For this review, use the dimensioned drawing (mm, ordinates from the lowest corner) and the shaded views. A direction names the side the tool comes from. Coordinates: 2 decimals unless noted, no trailing zeros. Loops run counter-clockwise (first coordinate to the right, second up) from the corner with the lowest first, then second, coordinate; pieces in that order, holes last. Notation, with made-up numbers: (58, -3.5) - (91, -3.5) arc R19 ccw to (91, 17.5) - close; hole circle Ø6 at (-4, 39). An arc over 180 degrees is marked (long way). Return JSON: item names as keys, results as strings. Group by question number.
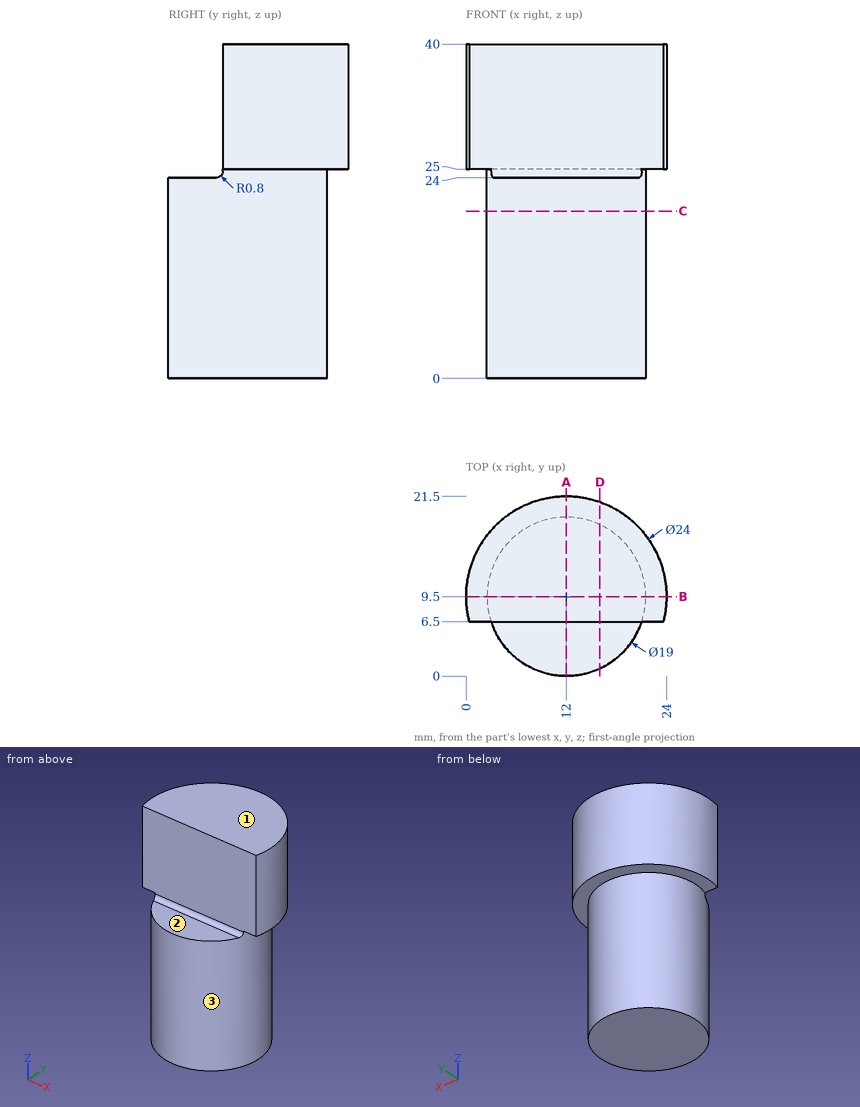
Item 1: To check wall thickness, follow line 1 (Z direction, x = 4.25, y = 17.25); line 2 (Z direction, x = 18, y = 5.25); line 3 (X direction, y = 17.75, z = 38). State the ranges of each line that lie inside material, in increasing order. Write a range as from..to.
Item 2: For the marked faces 1, 2 and 3, list the 3-axis set-ups (+Z, -Z, +X, -X, +Y, -Y) from which the entire face can be reached by the end or side of a thin tool; tool diameter is ignored.
Item 3: Add section C-C (z = 20). State the section outline as (x, y) points.
Item 4: Add section B-B (y = 9.5). State the section outline as (x, z) points, then the cut area to 3 significant figures.
Item 5: Add section D-D (x = 16). State the section outline as (y, z) points.
Item 6: Add section A-A (x = 12). State the section outline as (y, z) points, then the cut area to 3 significant figures.
Item 7: For P1, Ø12, axis at y = 7, z = 27, coming from the -X side; P2, Ø1, axis at x = 16, z = 22.5, coming from the +Y side; P3, Ø8, axis at x = 5.5, z = 24.5, coming from the +Y side; P4, Ø1, axis at x = 5.5, z = 13.5, coming from the -Y side, all flat-tipped, find the tip position at first contact; note any pin that passes through.
Answers below:
{
 "1": {"line 1": "z = 25..40", "line 2": "z = 0..24", "line 3": "x = 3.29..20.71"},
 "2": {"face 1": "+Z, +X, -X, +Y, -Y", "face 2": "+Z, +X, -X, -Y", "face 3": "-Z"},
 "3": {"outline": "circle Ø19 at (12, 9.5)"},
 "4": {"outline": "(0, 25) - (2.5, 25) - (2.5, 0) - (21.5, 0) - (21.5, 25) - (24, 25) - (24, 40) - (0, 40) - close", "area": "835 mm^2"},
 "5": {"outline": "(0.88, 0) - (18.12, 0) - (18.12, 25) - (20.81, 25) - (20.81, 40) - (6.5, 40) - (6.5, 24.8) arc R0.8 cw to (5.7, 24) - (0.88, 24) - close"},
 "6": {"outline": "(0, 0) - (19, 0) - (19, 25) - (21.5, 25) - (21.5, 40) - (6.5, 40) - (6.5, 24.8) arc R0.8 cw to (5.7, 24) - (0, 24) - close", "area": "694 mm^2"},
 "7": {"P1": "stops at x = 0", "P2": "stops at y = 18.33", "P3": "stops at y = 21.23", "P4": "stops at y = 2.13"}
}
